Geometry: final body of the model. Coordinates: model frame, mm. Coordinates: 2 decimals unless noted, no trailing zeros. Write each loop counter-clockwise with the first axis right and the second up, starting at its lowest first coordinate (ties: lowest second). Pieces come first, ordered by that corner, then holes. Notation, with made-up numbers: (61, 47.25) -> (75, 47.25) arc R18 cw to (75, 62.25) -> close; hole circle Ø9 at (56, 51.25). An arc over 180 degrees is marked (long way). Answer as a JSON object with one key per item and string values. Group by question number.
```python
from build123d import *

# Parameters (mm, degrees)
F0_W     = 141.0973854363
F0_H     = 69.7157457471
F1_DEPTH = 69.342
F3_DEPTH = 115.062
F5_DEPTH = 121.158


with BuildPart() as f1:
    # F0 (on Front) → F1 (new body)
    with BuildSketch(Plane.XZ):
        with Locations((13.8084646314, -22.6355418563)):
            Rectangle(F0_W, F0_H)
    extrude(amount=F1_DEPTH)

    # F2 (on face) → F3 (cut)
    with BuildSketch(Plane.XY.offset(12.2223310173)):
        Polygon((84.3571573496, -32.1864075959), (-56.7402280867, -69.342), (84.3571573496, -69.342), align=None)
    extrude(amount=-F3_DEPTH, mode=Mode.SUBTRACT)

    # F4 (on face) → F5 (cut)
    with BuildSketch(Plane.XY.offset(12.2223310173)):
        Polygon((84.3571573496, 0), (-56.7402280867, 0), (84.3571573496, -32.1864075959), align=None)
    extrude(amount=-F5_DEPTH, mode=Mode.SUBTRACT)


solid = f1.part
```
Item 1: Section B-B on x = 66. Output: boundary loops of the cut face in (y, z).
Item 2: Mould query, pull axis Y, two halves, no side actions, for faces 1 (the flat face through (14.796, -50.504, -22.148)), 2 (the flat face through (-3, -34, 12.222)), 3 (the flat face through (12.821, -15.868, -22.148)). Classes: +Y half, -Y half, draft (parallel to the pull), parting line (faces both ways), or undercut.
Item 3: Contact query for flat-ended pins moving along their axis: pin 1 (3 mm diameter, centred on x = 27.5, z = -8.5, fed in from +Y); pin 2 (3 mm diameter, centred on x = -27.5, z = -37, fed in from -Y); pin 3 (1 mm diameter, centred on x = -37.5, z = -3.5, fed in from -Y). Output: stop coordinate, or through.
Item 4: Section A-A on z = -14. Output: boundary loops of the cut face in (x, y).
Item 5: Ray query, L1, parallel to Y at x = 58, z = -9; L2, parallel to Y at x = 9, z = 2.5. Return the intervals inside material, ascending. Write a range as [from, to].
Item 6: Section C-C on y = -54. Output: boundary loops of the cut face in (x, z).
Answer sheet:
{
 "1": {"outline": "(-37.02, -57.49) -> (-28, -57.49) -> (-28, 12.22) -> (-37.02, 12.22) -> close"},
 "2": {"face 1": "-Y half", "face 2": "draft", "face 3": "+Y half"},
 "3": {"pin 1": "stops at y = -18.87", "pin 2": "stops at y = -62.04", "pin 3": "stops at y = -64.41"},
 "4": {"outline": "(-56.74, -69.34) -> (84.36, -32.19) -> (-56.74, 0) -> close"},
 "5": {"L1": "y = [-39.13, -26.17]", "L2": "y = [-52.03, -15]"},
 "6": {"outline": "(-56.74, -57.49) -> (1.52, -57.49) -> (1.52, 12.22) -> (-56.74, 12.22) -> close"}
}
